Verification items for the finished model (mm, model axes). Face numbers are marked on the shaded views. A direction names the side the tool comes from. Give positions to 0.01 mm unless a question says otherwise; leave off trailing zeros. Write each loop counter-clockwise with the first axis right and the second up, starting at its lowest first coordinate (ties: lowest second). Pieces come first, ordered by that corner, then holes. Notation, with made-up numbers: (-37.5, -36) -> (5.5, -36) arc R12 ccw to (5.5, -22) -> close; hole circle Ø10 at (14.25, 75). An arc over 180 degrees is marked (long way). Use one line per item in the form item = value. Start each with the question number.
(1) Release check for a two-part mould opening along X. For the marked faces 3, 4, 5 and 6 record: pulls with the +X half, pulls with the -X half, needs draft (parallel to the pull), parting line crosses it, or undercut.
(2) Scan lines: L1, parallel to Y at x = 22.5, z = -3.75; L2, parallel to X at y = -48.85, z = -10; L3, parallel to Y at x = 19, z = -8.5. Record each from-to range of solid material in increasing order.
(3) Depth check by flat-ended pin: pin 1 Ø8 at (x, z) = (30, -10) entering from -Y; pin 2 Ø5 at (x, z) = (30, -10) entering from +Y; pin 3 Ø1 at (y, z) = (-28, -10.5) entering from +X; pin 4 Ø5 at (x, y) = (8.5, -36) entering from +Z. Enter the tip coordinate at first touch or a pass-through.
(4) Section check D-D, the plane x = 24. Record the cut outline in (y, z), plus the area to 3 significant figures.
(5) Set-up check for the marked faces 1 and 2: record each of +Z, -Z, +X, -X, +Y, -Y from which the full face is reachable in a straight line by a thin tool's end or side.
(6) Section check A-A, the plane x = 10. Record the cut outline in (y, z), plus the area to 3 significant figures.
(7) Section check B-B, the plane z = -10. Record the cut outline in (x, y).
(8) Section check C-C, the plane z = -3. Record the cut outline in (x, y), plus the area to 3 significant figures.
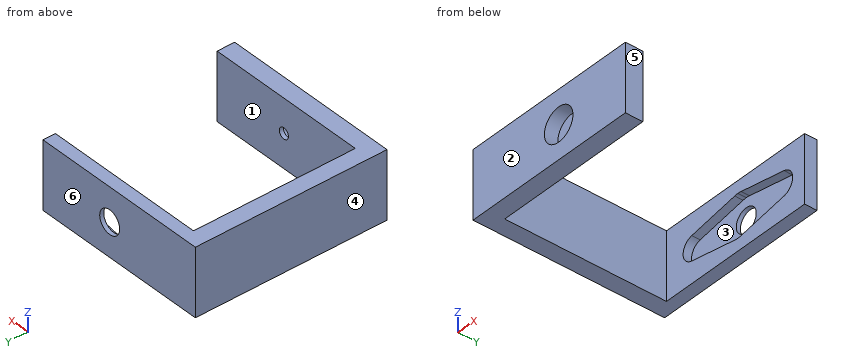
from build123d import *

# Parameters (mm, degrees)
CROQUIS1_W              = 53.36
CROQUIS1_H              = 20
SALIENTE_EXTRUIR1_DEPTH = 3.7
CROQUIS2_W              = 5
CROQUIS2_H              = 20
SALIENTE_EXTRUIR2_DEPTH = 48.17
CROQUIS3_W              = 53.36
CROQUIS3_H              = 20
SALIENTE_EXTRUIR3_DEPTH = 5.2
CORTAR_EXTRUIR1_DEPTH   = 2.5
CROQUIS5_R              = 3.5
CORTAR_EXTRUIR2_DEPTH   = 80.804426569
CROQUIS6_R              = 5
CORTAR_EXTRUIR3_DEPTH   = 4
CROQUIS7_R              = 1.6
CORTAR_EXTRUIR4_DEPTH   = 78.86985617


with BuildPart() as part:
    # Croquis1 → Saliente-Extruir1 (new body)
    with BuildSketch(Plane(origin=(0, 0, 0), x_dir=(1, 0, 0), z_dir=(0, 1, 0))):
        with Locations((26.68, 10)):
            Rectangle(CROQUIS1_W, CROQUIS1_H)
    extrude(amount=SALIENTE_EXTRUIR1_DEPTH)

    # Croquis2 → Saliente-Extruir2 (add)
    with BuildSketch(Plane.XZ):
        with Locations((2.5, -10)):
            Rectangle(CROQUIS2_W, CROQUIS2_H)
    extrude(amount=SALIENTE_EXTRUIR2_DEPTH)

    # Croquis3 → Saliente-Extruir3 (add)
    with BuildSketch(Plane.XZ.offset(48.17)):
        with Locations((26.68, -10)):
            Rectangle(CROQUIS3_W, CROQUIS3_H)
    extrude(amount=SALIENTE_EXTRUIR3_DEPTH)

    # Croquis4 → Cortar-Extruir1 (cut)
    with BuildSketch(Plane.XZ):
        with BuildLine():
            Line((28.897334072, -3.746470768), (13.839427952, -6.40158589))
            ThreePointArc((13.839427952, -6.40158589), (10.82, -10), (13.839427952, -13.59841411))
            Line((13.839427952, -13.59841411), (28.897334072, -16.253529232))
            ThreePointArc((28.897334072, -16.253529232), (29.446561034, -16.325836333), (30, -16.35))
            Line((30, -16.35), (30, -3.65))
            ThreePointArc((30, -3.65), (29.446561034, -3.674163667), (28.897334072, -3.746470768))
        make_face()
    cortar_extruir1 = extrude(amount=-CORTAR_EXTRUIR1_DEPTH, mode=Mode.SUBTRACT)

    # Simetría1: Cortar-Extruir1 across plane
    add(cortar_extruir1.mirror(Plane(origin=(30, 2.5, -3.65), x_dir=(0, 0, 1), z_dir=(1, 0, 0))), mode=Mode.SUBTRACT)

    # Croquis5 → Cortar-Extruir2 (cut, through all)
    with BuildSketch(Plane.XZ.offset(-2.5)):
        with Locations(Location((30, -10, 0), (0, 0, 270))):
            Circle(CROQUIS5_R)
    extrude(amount=-CORTAR_EXTRUIR2_DEPTH, mode=Mode.SUBTRACT)

    # Croquis6 → Cortar-Extruir3 (cut)
    with BuildSketch(Plane.XZ.offset(53.37)):
        with Locations(Location((30, -10, 0), (0, 0, 270))):
            Circle(CROQUIS6_R)
    extrude(amount=-CORTAR_EXTRUIR3_DEPTH, mode=Mode.SUBTRACT)

    # Croquis7 → Cortar-Extruir4 (cut, through all)
    with BuildSketch(Plane.XZ.offset(49.37)):
        with Locations(Location((30, -10, 0), (0, 0, 270))):
            Circle(CROQUIS7_R)
    extrude(amount=-CORTAR_EXTRUIR4_DEPTH, mode=Mode.SUBTRACT)


solid = part.part
Completed:
q1.face_3 = undercut
q1.face_4 = pulls with the -X half
q1.face_5 = pulls with the +X half
q1.face_6 = needs draft
q2.L1 = -53.37 to -48.17, 0 to 3.7
q2.L2 = 0 to 28.4, 31.6 to 53.36
q2.L3 = -53.37 to -48.17, 2.5 to 3.7
q3.pin_1 = -49.37
q3.pin_2 = -48.17
q3.pin_3 = 5
q3.pin_4 = through
q4.outline = (-53.37, -20) -> (-48.17, -20) -> (-48.17, 0) -> (-53.37, 0) -> close; (0, -20) -> (3.7, -20) -> (3.7, 0) -> (0, 0) -> (0, -4.61) -> (2.5, -4.61) -> (2.5, -15.39) -> (0, -15.39) -> close
q4.area = 151 mm²
q5.face_1 = +Z, -Z, +X
q5.face_2 = +Z, -Z, +X, -X, -Y
q6.outline = (-53.37, -20) -> (-48.17, -20) -> (-48.17, 0) -> (-53.37, 0) -> close; (0, -20) -> (3.7, -20) -> (3.7, 0) -> (0, 0) -> close
q6.area = 178 mm²
q7.outline = (0, -53.37) -> (25, -53.37) -> (25, -49.37) -> (28.4, -49.37) -> (28.4, -48.17) -> (5, -48.17) -> (5, 0) -> (10.82, 0) -> (10.82, 2.5) -> (26.5, 2.5) -> (26.5, 3.7) -> (0, 3.7) -> close; (31.6, -49.37) -> (35, -49.37) -> (35, -53.37) -> (53.36, -53.37) -> (53.36, -48.17) -> (31.6, -48.17) -> close; (33.5, 2.5) -> (49.18, 2.5) -> (49.18, 0) -> (53.36, 0) -> (53.36, 3.7) -> (33.5, 3.7) -> close
q8.outline = (0, -53.37) -> (53.36, -53.37) -> (53.36, -48.17) -> (5, -48.17) -> (5, 0) -> (53.36, 0) -> (53.36, 3.7) -> (0, 3.7) -> close
q8.area = 716 mm²
